Read the model definition and answer for the solid it produces. Units are mm, in the model's axes. A direction names the side the tool comes from. Give positions to 0.01 mm unless a question says otherwise; leave off trailing zeros. Order: outer loops, then holes, each group sorted by start corner. A loop starts at its lowest first (then second) coordinate and runs counter-clockwise, first axis right, second up.
```python
from build123d import *

# Parameters (mm, degrees)
F0_W     = 60
F0_H     = 30
F0_R     = 2
F0_R_2   = 12
F1_DEPTH = 25
F2_D     = 4.5
F3_DEPTH = 20


with BuildPart() as f1:
    # F0 (on Top) → F1 (new body)
    with BuildSketch(Plane.XY):
        with Locations((0, 0.1760203019)):
            Rectangle(F0_W, F0_H)
        with Locations((-25, -9.8239796981)):
            Circle(F0_R, mode=Mode.SUBTRACT)
        with Locations((25, -9.8239796981)):
            Circle(F0_R, mode=Mode.SUBTRACT)
        with Locations((0, 0.1760203019)):
            Circle(F0_R_2, mode=Mode.SUBTRACT)
        with Locations((-25, 10.1760203019)):
            Circle(F0_R, mode=Mode.SUBTRACT)
        with Locations((25, 10.1760203019)):
            Circle(F0_R, mode=Mode.SUBTRACT)
        with Locations((0, 0.1760203019)):
            Circle(F0_R_2)
        with BuildLine():
            ThreePointArc((-2.5620431112, -6.3382666964), (0.0664242114, 7.1757051394), (2.4379568888, -6.385714698))
            Line((2.4379568888, -6.385714698), (2.4379568888, -9.3239796981))
            Line((2.4379568888, -9.3239796981), (-2.5620431112, -9.3239796981))
            Line((-2.5620431112, -9.3239796981), (-2.5620431112, -6.3382666964))
        make_face(mode=Mode.SUBTRACT)
    extrude(amount=F1_DEPTH)

    # F2 (through all)
    with Locations(Plane(origin=(0, 0, 0), x_dir=(1, 0, 0), z_dir=(0, 0, -1))):
        with Locations((-25, 9.8239796981), (-25, -10.1760203019), (25, -10.1760203019), (25, 9.8239796981)):
            Hole(F2_D / 2)

    # F0 (on Top) → F3 (cut)
    with BuildSketch(Plane.XY):
        with Locations((0, 0.1760203019)):
            Rectangle(F0_W, F0_H)
        with Locations((-25, -9.8239796981)):
            Circle(F0_R, mode=Mode.SUBTRACT)
        with Locations((25, -9.8239796981)):
            Circle(F0_R, mode=Mode.SUBTRACT)
        with Locations((0, 0.1760203019)):
            Circle(F0_R_2, mode=Mode.SUBTRACT)
        with Locations((-25, 10.1760203019)):
            Circle(F0_R, mode=Mode.SUBTRACT)
        with Locations((25, 10.1760203019)):
            Circle(F0_R, mode=Mode.SUBTRACT)
    extrude(amount=F3_DEPTH, mode=Mode.SUBTRACT)


solid = f1.part
```
1) Consider L1, parallel to Y at x = -25, z = 21.05; L2, parallel to X at y = 11.5, z = 23.25; L3, parallel to X at y = -0.25, z = 7.75. Determine where each line is inside the solid, lowest interval first.
Final values:
L1: y = -14.82 to -12.07, -7.57 to 7.93, 12.43 to 15.18
L2: x = -30 to -26.82, -23.18 to 23.18, 26.82 to 30
L3: x = -11.99 to -6.99, 6.99 to 11.99
2) The part is cut by section C-C on x = -25. Determine the outline of the cut face in (y, z).
Final values:
outline: (-14.82, 20) - (-12.07, 20) - (-12.07, 25) - (-14.82, 25) - close; (-7.57, 20) - (7.93, 20) - (7.93, 25) - (-7.57, 25) - close; (12.43, 20) - (15.18, 20) - (15.18, 25) - (12.43, 25) - close
3) For a pull along X with two mould halves and no side action, classify faces 3 (the face through (-9.52, -7.13, 9.86)), 4 (the face through (-7.1, 10.4, 20)), 5 (the face through (-27.146, -10.5, 22.535)) as released by +X, released by -X, zero draft, split by the parting line, or undercut.
Final values:
face 3: split by the parting line
face 4: zero draft
face 5: undercut
4) The part is cut by section D-D on y = 2.25. Determine the outline of the cut face in (x, z).
Final values:
outline: (-30, 20) - (-11.82, 20) - (-11.82, 0) - (-6.69, 0) - (-6.69, 25) - (-30, 25) - close; (6.69, 0) - (11.82, 0) - (11.82, 20) - (30, 20) - (30, 25) - (6.69, 25) - close
5) Given pin 1 (6 mm diameter, centred on x = -25, y = -9.82, fed in from +Z); pin 2 (2 mm diameter, centred on y = 2, z = 5.5, fed in from -X); pin 3 (1.5 mm diameter, centred on y = -7.5, z = 16, fed in from +X); pin 4 (2.5 mm diameter, centred on y = -8, z = 18.5, fed in from -X), each flat-ended and moving along its own axis, determine where each tip first touches the part or whether it passes through.
Final values:
pin 1: stops at z = 25
pin 2: stops at x = -11.97
pin 3: stops at x = 9.8
pin 4: stops at x = -9.8
6) A tool of negligible diameter and unlimited length cuts with its end or side. For faces 1 (the face through (-2.562, -8, 12)), 2 (the face through (0, 15.176, 22)), from which of +Z, -Z, +X, -X, +Y, -Y can it reach the whole face along a straight path? Write none if from no direction.
Final values:
face 1: +Z, -Z
face 2: +Z, -Z, +X, -X, +Y
7) The part is cut by section A-A on x = 0. Determine the outline of the cut face in (y, z).
Final values:
outline: (-14.82, 20) - (-11.82, 20) - (-11.82, 0) - (-9.32, 0) - (-9.32, 25) - (-14.82, 25) - close; (7.18, 0) - (12.18, 0) - (12.18, 20) - (15.18, 20) - (15.18, 25) - (7.18, 25) - close
8) The part is cut by section B-B on y = -10.5. Determine the outline of the cut face in (x, z), and give its area (3 significant figures).
Final values:
outline: (-30, 20) - (-27.15, 20) - (-27.15, 25) - (-30, 25) - close; (-22.85, 20) - (-5.48, 20) - (-5.48, 0) - (5.48, 0) - (5.48, 20) - (22.85, 20) - (22.85, 25) - (-22.85, 25) - close; (27.15, 20) - (30, 20) - (30, 25) - (27.15, 25) - close
area: 476 mm2
